Work out the finished part from the listing and answer in its coordinate system (mm). Face numbers are marked on the shaded views. A direction names the side the tool comes from. Coordinates: 2 decimals unless noted, no trailing zeros. Order: outer loops, then holes, each group sorted by start corner. A loop starts at its lowest first (then second) coordinate and runs counter-clockwise, first axis right, second up.
Autodesk Inventor part; units mm, degrees
ref_plane "YZ Plane" through (0, 0, 0) normal (1, 0, 0) x (0, 1, 0)
ref_plane "XZ Plane" through (0, 0, 0) normal (0, 1, 0) x (-1, 0, 0)
ref_plane "XY Plane" through (0, 0, 0) normal (0, 0, 1) x (1, 0, 0)
sketch "Sketch1" plane through (0, 0, 0) normal (0, 0, 1) x (1, 0, 0)
  line L0 (-12.7, 12.7) -> (12.7, 12.7)
  line L1 (12.7, 12.7) -> (12.7, -12.7)
  line L2 (12.7, -12.7) -> (-12.7, -12.7)
  line L3 (-12.7, -12.7) -> (-12.7, 12.7)
  line L4 (-9.525, 9.525) -> (9.525, 9.525)
  line L5 (9.525, 9.525) -> (9.525, -9.525)
  line L6 (9.525, -9.525) -> (-9.525, -9.525)
  line L7 (-9.525, -9.525) -> (-9.525, 9.525)
  point P0 (0, 0)
  dimension "d0" = 25.4
  dimension "d1" = 25.4
  dimension "d2" = 12.7
  dimension "d3" = 12.7
  dimension "d4" = 3.175
  dimension "d5" = 3.175
  dimension "d6" = 3.175
  dimension "d7" = 3.175
extrude "Extrusion1" add sketch "Sketch1" along normal blind 180.975
sketch "Sketch3" plane through (-12.7, 12.7, 0) normal (0, 1, 0) x (1, 0, 0)
  line L0 (0, -180.975) -> (25.4, -180.975)
  line L1 (25.4, 0) -> (25.4, -180.975)
  line L2 (0, 0) -> (0, -180.975)
  line L3 (0, -180.975) -> (25.4, -155.575)
  point P0 (12.7, 0)
  dimension "d13" = 45
extrude "Extrusion3" cut sketch "Sketch3" against normal blind 25.4
properties part number "backwards edge frame tube"
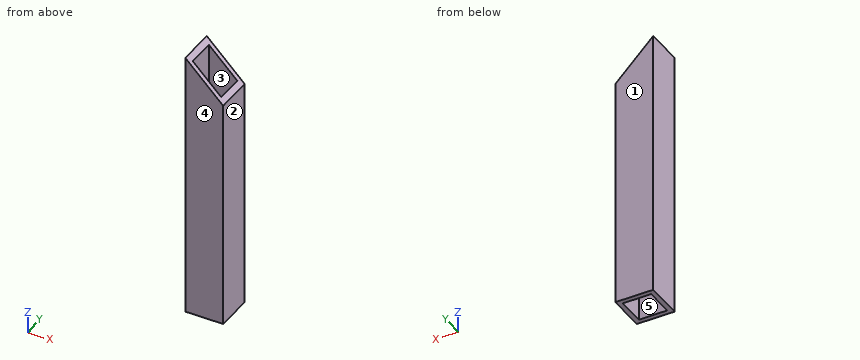
1. The mould has two halves that part along Y. Classify the marked faces 1, 2 and 3: released by +Y, released by -Y, zero draft, split by the parting line, or undercut.
2. The part is cut by section C-C (z = 144). Determine the outline of the cut face in (x, y) (3 decimals).
3. A flat-ended cylindrical pin translates along its axis: pin 1 (8 mm diameter, centred on x = -8, y = -4, fed in from +Z) (3 decimals). Find the tip coordinate at first contact, or state that the pin passes through.
4. The part is cut by section A-A (y = -4.5). Determine the outline of the cut face in (x, z) (3 decimals).
5. The part is cut by section B-B (x = 0.25). Determine the outline of the cut face in (y, z) (3 decimals).
6. Consider probe 1 along X at (y, z) = (7.5, 128) (3 decimals); probe 2 along X at (y, z) = (5.25, 170.5) (3 decimals). Determine where each line is inside the solid, lowest interval first.
7. For the marked faces 4 and 5, determine the directions among +Z, -Z, +X, -X, +Y, -Y from which every point of the face is accessible in a straight line to the end or side of a thin tool.
Worked out:
1. face 1: released by +Y
1. face 2: zero draft
1. face 3: undercut
2. outline: (-12.7, -12.7) - (12.7, -12.7) - (12.7, 12.7) - (-12.7, 12.7) - close; hole (-9.525, -9.525) - (9.525, -9.525) - (9.525, 9.525) - (-9.525, 9.525) - close
3. pin 1: stops at z = 180.275
4. outline: (-12.7, 0) - (-9.525, 0) - (-9.525, 177.8) - (-12.7, 180.975) - close; (9.525, 0) - (12.7, 0) - (12.7, 155.575) - (9.525, 158.75) - close
5. outline: (-12.7, 0) - (-9.525, 0) - (-9.525, 168.025) - (-12.7, 168.025) - close; (9.525, 0) - (12.7, 0) - (12.7, 168.025) - (9.525, 168.025) - close
6. probe 1: x = -12.7 to -9.525, 9.525 to 12.7
6. probe 2: x = -12.7 to -9.525
7. face 4: +Z, -Z, +X, -X, -Y
7. face 5: +Z, -Z
